Could you check a few things on this model? Use its own coordinates, in mm. A direction names the side the tool comes from. Give positions to 0.01 mm unless a question says otherwise; leave off trailing zeros. Loops run counter-clockwise (first coordinate to the right, second up) from the corner with the lowest first, then second, coordinate; pieces in that order, holes last. Notation, with made-up numbers: (43.25, 86) - (57.25, 86) arc R20 cw to (57.25, 94) - close; hole circle Ø8 at (33.5, 45.5). An arc over 180 degrees is marked (long way). Use CSV: the item, a comma, the result in double quotes.
from build123d import *

# Parameters (mm, degrees)
BOSS_EXTRUDE1_DEPTH = 5
BOSS_EXTRUDE2_DEPTH = 5
FILLET1_R           = 5
SKETCH3_R           = 5.5
SKETCH3_R_2         = 2.15
BOSS_EXTRUDE3_DEPTH = 8
SKETCH4_R           = 2.15
CUT_EXTRUDE1_DEPTH  = 6


with BuildPart() as part:
    # Sketch1 → Boss-Extrude1 (new body)
    with BuildSketch(Plane.XY):
        with BuildLine():
            Line((0, 8), (180, 8))
            ThreePointArc((180, 8), (188, 0), (180, -8))
            Line((180, -8), (0, -8))
            ThreePointArc((0, -8), (-8, 0), (0, 8))
        make_face()
        with BuildLine():
            Line((175.411388509, 6.553216354), (224.560511167, 40.967802535))
            ThreePointArc((224.560511167, 40.967802535), (235.702339012, 39.003197672), (233.737734148, 27.861369827))
            Line((233.737734148, 27.861369827), (184.588611491, -6.553216354))
            ThreePointArc((184.588611491, -6.553216354), (173.446783646, -4.588611491), (175.411388509, 6.553216354))
        make_face()
        with BuildLine():
            Line((225.149122657, 27.486382951), (164.527344392, 62.486382951))
            ThreePointArc((164.527344392, 62.486382951), (161.599141162, 73.414586181), (172.527344392, 76.342789411))
            Line((172.527344392, 76.342789411), (233.149122657, 41.342789411))
            ThreePointArc((233.149122657, 41.342789411), (236.077325888, 30.414586181), (225.149122657, 27.486382951))
        make_face()
        with BuildLine():
            Line((-3.04678556, 7.397100632), (165.480558833, 76.811686813))
            ThreePointArc((165.480558833, 76.811686813), (175.924445024, 72.461371741), (171.574129952, 62.017485549))
            Line((171.574129952, 62.017485549), (3.04678556, -7.397100632))
            ThreePointArc((3.04678556, -7.397100632), (-7.397100632, -3.04678556), (-3.04678556, 7.397100632))
        make_face()
    extrude(amount=BOSS_EXTRUDE1_DEPTH)

    # Sketch2 → Boss-Extrude2 (add)
    with BuildSketch(Plane.XY.offset(5)):
        Polygon((147.229345289, 8), (175.147140962, 56.355040542), (167.935409097, 60.518735876), (157.826632887, 56.355040542), (129.908837213, 8), align=None)
    extrude(amount=-BOSS_EXTRUDE2_DEPTH)

    # Fillet1
    fillet1_edges = [part.edges().sort_by_distance(p)[0] for p in [
        (40.428445864, 8, 2.5),
        (177.477609689, 8, 2.5),
        (214.274021971, 33.765125259, 2.5),
        (157.826632887, 56.355040542, 2.5),
        (129.908837213, 8, 2.5),
        (147.229345289, 8, 2.5),
        (175.147140962, 56.355040542, 2.5),
    ]]
    fillet(fillet1_edges, radius=FILLET1_R)

    # Sketch3 → Boss-Extrude3 (add)
    with BuildSketch(Plane.XY.offset(5)):
        with Locations((174.937796577, 64.5)):
            Circle(SKETCH3_R)
        with Locations((174.937796577, 64.5)):
            Circle(SKETCH3_R_2, mode=Mode.SUBTRACT)
        with Locations((229.149122657, 34.414586181)):
            Circle(SKETCH3_R)
        with Locations((229.149122657, 34.414586181)):
            Circle(SKETCH3_R_2, mode=Mode.SUBTRACT)
        with Locations((176.018340463, 1.5)):
            Circle(SKETCH3_R)
        with Locations((176.018340463, 1.5)):
            Circle(SKETCH3_R_2, mode=Mode.SUBTRACT)
        with Locations((120.218340463, 1.5)):
            Circle(SKETCH3_R)
        with Locations((120.218340463, 1.5)):
            Circle(SKETCH3_R_2, mode=Mode.SUBTRACT)
        with Locations((65.018340463, 1.5)):
            Circle(SKETCH3_R)
        with Locations((65.018340463, 1.5)):
            Circle(SKETCH3_R_2, mode=Mode.SUBTRACT)
        with Locations((9.018340463, 1.5)):
            Circle(SKETCH3_R)
        with Locations((9.018340463, 1.5)):
            Circle(SKETCH3_R_2, mode=Mode.SUBTRACT)
    extrude(amount=BOSS_EXTRUDE3_DEPTH)

    # Sketch4 → Cut-Extrude1 (cut, through all)
    with BuildSketch(Plane.XY.offset(5)):
        with Locations((9.018340463, 1.5)):
            Circle(SKETCH4_R)
        with Locations((65.018340463, 1.5)):
            Circle(SKETCH4_R)
        with Locations((120.218340463, 1.5)):
            Circle(SKETCH4_R)
        with Locations((176.018340463, 1.5)):
            Circle(SKETCH4_R)
        with Locations((229.149122657, 34.414586181)):
            Circle(SKETCH4_R)
        with Locations((174.937796577, 64.5)):
            Circle(SKETCH4_R)
    extrude(amount=-CUT_EXTRUDE1_DEPTH, mode=Mode.SUBTRACT)


solid = part.part
1) Which directions (+Z, -Z, +X, -X, +Y, -Y) give clear straight access to the entire face, cutting with the end or side of a thin tool? Please do faces 4 (the cylindrical face through (129.554, 8.688, 2.465)), 5 (the cylindrical face through (181.264, 3.152, 8.944)), 6 (the cylindrical face through (169, 77.4, 2.5)).
Answer below:
face 4,"+Z, -Z"
face 5,"+Z"
face 6,"+Z, -Z, +Y"
2) Suppose I cut it at D-D (x = 136). Please give me the cut outline in (y, z).
Answer below:
outline,"(-8, 0) - (18.55, 0) - (18.55, 5) - (-8, 5) - close; (47.36, 0) - (64.67, 0) - (64.67, 5) - (47.36, 5) - close"
3) I need wall thicknesses on line 1 along X through (y, z) = (31, 4.25); line 2 along Z through (x, y) = (162, -1.5); line 3 along X through (y, z) = (20, 3.5). Which ranges of each line are inside material? Lowest first, please.
Answer below:
line 1,"x = 54.26 to 96.27, 143.19 to 160.51, 209.39 to 236.38"
line 2,"z = 0 to 5"
line 3,"x = 27.55 to 69.56, 136.84 to 154.16, 194.62 to 222.51"
4) I'm going to push flat-ended pins straight in: P1, Ø1, axis at y = 12, z = 6, coming from the +X side; P2, Ø1.5, axis at x = 117, y = 52, coming from the +Z side; P3, Ø4, axis at y = 5.5, z = 8.5, coming from the +X side; P4, Ø5.5, axis at x = 97.5, z = 1.5, coming from the +Y side. Where does each tip first touch, or does it pass through?
Answer below:
P1,"passes through"
P2,"stops at z = 5"
P3,"stops at x = 181.14"
P4,"stops at y = 49.94"
5) We'd pull the mould along X, two halves only. Please class faces 1 (the flat face through (120, -1, 13)), 2 (the flat face through (80.04, 41.62, 2.46)), 3 (the flat face through (113, 7, 5)): +X half, -X half, draft (parallel to the pull), parting line (faces both ways), or undercut.
Answer below:
face 1,"draft"
face 2,"-X half"
face 3,"undercut"
6) Suppose I cut it at A-A (z = 8.25). State how many separate pieces and enclosed holes the cut face has, plus the area to 3 significant figures.
Answer below:
separate pieces,"6"
enclosed holes,"6"
area,"483 mm2"
7) Suppose I cut it at B-B (x = 106). Please give me the cut outline in (y, z).
Answer below:
outline,"(-8, 0) - (8, 0) - (8, 5) - (-8, 5) - close; (35.01, 0) - (52.31, 0) - (52.31, 5) - (35.01, 5) - close"
8) Suppose I cut it at C-C (y = 64.5). Please give me the cut outline in (x, z).
Answer below:
outline,"(135.59, 0) - (172.79, 0) - (172.79, 13) - (169.44, 13) - (169.44, 5) - (135.59, 5) - close; (177.09, 0) - (193.04, 0) - (193.04, 5) - (180.44, 5) - (180.44, 13) - (177.09, 13) - close"
